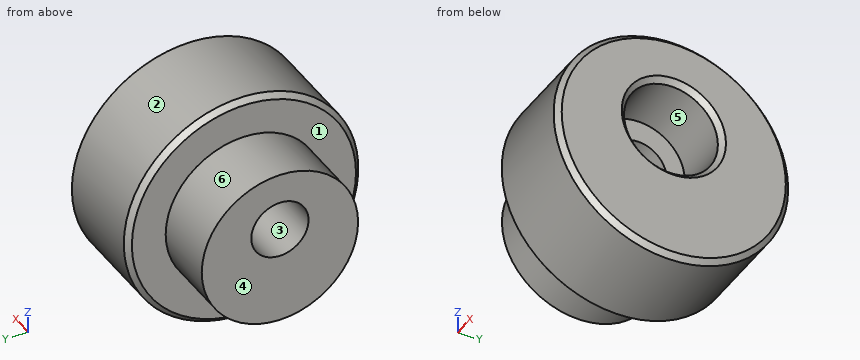
from build123d import *

# Parameters (mm, degrees)
SKETCH005_R             = 6
SKETCH005_R_2           = 2.2
PAD002_DEPTH            = 5
SKETCH006_R             = 9
SKETCH006_R_2           = 2.2
PAD003_DEPTH            = 8
SKETCH007_R             = 3.6
POCKET_DEPTH            = 5
CHAMFER002_SIZE         = 0.4
BODY002_PLACEMENT_ANGLE = 90


with BuildPart() as part:
    # Sketch005 → Pad002 (new body)
    with BuildSketch(Plane.XZ):
        with Locations((66.64711, 33.3637672875)):
            Circle(SKETCH005_R)
        with Locations((66.64711, 34.8637672875)):
            Circle(SKETCH005_R_2, mode=Mode.SUBTRACT)
    extrude(amount=PAD002_DEPTH)

    # Sketch006 (on Face4 of Pad002) → Pad003 (join)
    with BuildSketch(Plane.XZ.offset(5)):
        with Locations((66.641708, 33.373905)):
            Circle(SKETCH006_R)
        with Locations((66.641708, 34.873905)):
            Circle(SKETCH006_R_2, mode=Mode.SUBTRACT)
    extrude(amount=PAD003_DEPTH)

    # Sketch007 (on Face8 of Pad003) → Pocket (cut)
    with BuildSketch(Plane.XZ.offset(13)):
        with Locations((66.648621, 35.148872)):
            Circle(SKETCH007_R)
    extrude(amount=-POCKET_DEPTH, mode=Mode.SUBTRACT)

    # Chamfer002
    chamfer002_edges = [part.edges().sort_by_distance(p)[0] for p in [
        (57.641708, -13, 33.373905),
        (57.641708, -5, 33.373905),
        (63.048621, -13, 35.148872),
    ]]
    chamfer(chamfer002_edges, length=CHAMFER002_SIZE)


with BuildPart() as part_1:
    # Body001 placement: moved
    add(part.part.moved(Location((0, -3, 0))))


with BuildPart() as part_2:
    # Clone placement: moved
    add(part_1.part.moved(Location((0, 3, 0))))


with BuildPart() as part_3:
    # Body002 placement: moved
    add(part_2.part.moved(Location((94, -15.33, -2.61))).rotate(Axis((94, -15.33, -2.61), (0, 0, 1)), BODY002_PLACEMENT_ANGLE))


solid = part_3.part
Can you work these out from the model? Positions are in its coordinate system, mm. Face numbers are marked on the shaded views. A direction names the side the tool comes from. Coordinates: 2 decimals unless noted, no trailing zeros. Write each loop counter-clockwise with the first axis right and the second up, starting at its lowest first coordinate (ties: lowest second). Pieces come first, ordered by that corner, then holes. Notation, with made-up numbers: (7, 1.5) - (30, 1.5) arc R14 ccw to (30, 14.5) - close; hole circle Ø5 at (50.5, 20). An arc over 180 degrees is marked (long way). Return JSON: item names as keys, results as strings. Group by question number.
Item 1: If we section it at A-A (x = 95.25): Write out the boundary of the cut face in (y, z).
Item 2: I'm going to push flat-ended pins straight in: pin 1 Ø5 at (x, z) = (102, 24.5) entering from -Y; pin 2 Ø3.5 at (y, z) = (52, 32.5) entering from +X; pin 3 Ø1 at (x, y) = (103, 47) entering from +Z. Where does each tip first touch, or does it pass through?
Item 3: Please list where these lines run through material, in increasing order: probe 1 along X at (y, z) = (48.5, 33.25); probe 2 along Z at (x, y) = (106.5, 48.25); probe 3 along Z at (x, y) = (102.5, 53.5).
Item 4: Which directions (+Z, -Z, +X, -X, +Y, -Y) give clear straight access to the entire face, cutting with the end or side of a thin tool? Please do the marked faces 4, 5 and 6.
Item 5: We'd pull the mould along Z, two halves only. Please class the marked faces 1, 2 and 3: pulls with the +Z half, pulls with the -Z half, needs draft (parallel to the pull), parting line crosses it, or undercut.
Item 6: If we section it at B-B (x = 105.5): Write out the boundary of the cut face in (y, z), then the cut area to 3 significant figures.
Return value:
{
 "1": {"outline": "circle Ø12 at (51.32, 30.75); hole circle Ø4.4 at (51.32, 32.25)"},
 "2": {"pin 1": "stops at y = 43.14", "pin 2": "stops at x = 102", "pin 3": "stops at z = 38.92"},
 "3": {"probe 1": "x = 94 to 102", "probe 2": "z = 22.3 to 30.66, 34.42 to 39.23", "probe 3": "z = 22.03 to 29.68, 35.4 to 39.49"},
 "4": {"face 4": "+Z, -Z, -X, +Y, -Y", "face 5": "+X", "face 6": "-X"},
 "5": {"face 1": "needs draft", "face 2": "parting line crosses it", "face 3": "undercut"},
 "6": {"outline": "circle Ø18 at (51.31, 30.76); hole circle Ø7.2 at (51.32, 32.54)", "area": "214 mm^2"}
}
